For this review, use the dimensioned drawing (mm, ordinates from the lowest corner) and the shaded views. A direction names the side the tool comes from. Round coordinates to 2 decimals unless told otherwise and drop trailing zeros. Order: outer loops, then holes, each group sorted by start corner. A loop starts at its lowest first (then second) coordinate and runs counter-clockwise, first axis right, second up. Notation, with made-up numbers: M 55,34.5 L 100,34.5 A22 cw 100,63.5 Z; hole C 22,9.5 d4. An arc over 180 degrees is marked long. One line per item, written item: value. Start each with the question number.
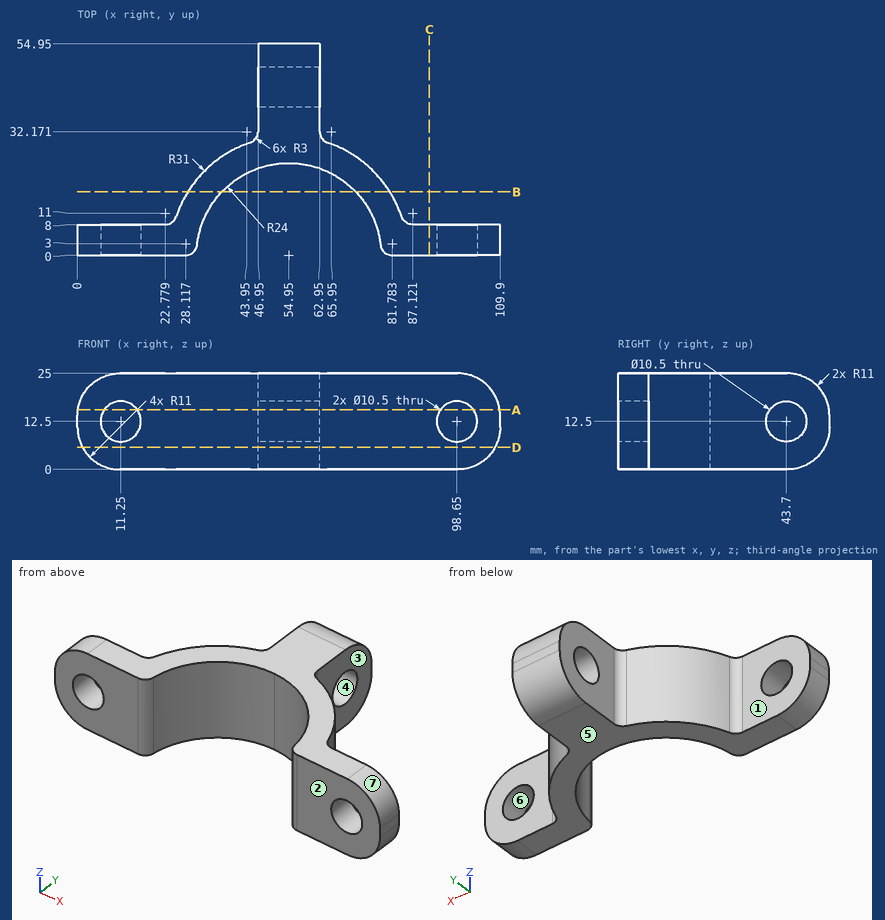
Item 1: Machinability: for the marked faces 1, 2 and 3, which of the approach directions +Z, -Z, +X, -X, +Y, -Y give a long, thin tool a straight path to every point of the face, cutting with its end or side? Answer none if there is none.
Item 2: Consider section C-C, the plane x = 91.5. Give the boundary of the cut face in (y, z).
Item 3: Wall thickness on L1, parallel to Z at x = 11, y = 3 (1 decimal); L2, parallel to X at y = 19.5, z = 12; L3, parallel to X at y = 7, z = 17 (1 decimal): over which ranges is each line inside the solid? List them lowest first.
Item 4: The part is to be moulded in two halves that separate along Z. For the marked faces 4, 5, 6 and 7, say which applies: pulls with the +Z half, pulls with the -Z half, needs draft (parallel to the pull), parting line crosses it, or undercut.
Item 5: Consider section B-B, the plane y = 16.5. Give the boundary of the cut face in (x, z) (1 decimal), then the cut area to 3 significant figures.
Item 6: Consider section A-A, the plane z = 15.5. Count the separate pieces of the cut face and the enclosed holes in it, then the cut area to 3 significant figures.
Item 7: Consider section D-D, the plane z = 5.75. Give the boundary of the cut face in (x, y).
Item 8: Clearance check with flat-ended pins moving along their axes: P1, Ø1, axis at x = 50.5, z = 6, coming from the +Y side; P2, Ø1, axis at x = 42, z = 20, coming from the -Y side; P3, Ø6.5, axis at y = 43.7, z = 12.5, coming from the -X side; P4, Ø11.5, axis at x = 6, z = 9.5, coming from the +Y side. State where each tip first meets the part, or that it passes through.
Computed:
1. face 1: +Z, -Z, -X, +Y
1. face 2: +Z, -Z, +X, -X, -Y
1. face 3: +Z, -Z, +X, +Y
2. outline: M 0,0 L 8,0 L 8,25 L 0,25 Z
3. L1: z = 0 to 7.3, 17.7 to 25
3. L2: x = 30.85 to 40.96, 68.94 to 79.05
3. L3: x = 0.4 to 8.5, 14 to 32, 77.9 to 95.9, 101.4 to 109.5
4. face 4: undercut
4. face 5: pulls with the -Z half
4. face 6: undercut
4. face 7: pulls with the +Z half
5. outline: M 28.7,0 L 37.5,0 L 37.5,25 L 28.7,25 Z; M 72.4,0 L 81.2,0 L 81.2,25 L 72.4,25 Z
5. area: 441 mm^2
6. separate pieces: 4
6. enclosed holes: 0
6. area: 1,100 mm^2
7. outline: M 1.33,0 L 28.12,0 A3 ccw 31.1,2.67 A24 cw 54.95,24 A24 cw 78.8,2.67 A3 ccw 81.78,0 L 108.57,0 L 108.57,8 L 87.12,8 A3 cw 84.28,10.03 A31 ccw 64.98,29.33 A3 cw 62.95,32.17 L 62.95,53.62 L 46.95,53.62 L 46.95,32.17 A3 cw 44.92,29.33 A31 ccw 25.62,10.03 A3 cw 22.78,8 L 1.33,8 Z
8. P1: stops at y = 53.99
8. P2: stops at y = 19.88
8. P3: passes through
8. P4: stops at y = 8
